The model under review builds one solid part; all positions refer to its coordinate system, in mm. Face numbers are marked on the shaded views. Give positions to 0.01 mm unless a question says otherwise; leave off trailing zeros. Loops run counter-clockwise (first coordinate to the right, second up) from the corner with the lowest first, then second, coordinate; pieces in that order, holes last. Notation, with made-up numbers: M 23,85.5 L 44,85.5 A38 cw 44,123.5 Z; hole C -20,71.5 d10. An arc over 180 degrees is marked long. Write item = value, one per line. Start each with the question number.
1. We need section B-B on y = 0. Give the boundary of the cut face in (x, z).
2. We need section D-D on x = 2.25. Give the boundary of the cut face in (y, z).
3. Draft analysis for pull direction Y (two halves, no side actions). For the marked faces 1, 2, 3 and 4, state which applies: pulls with the +Y half, pulls with the -Y half, needs draft (parallel to the pull), parting line crosses it, or undercut.
4. Wall thickness on line 1 along Y through (x, z) = (-0.5, 0.35); line 2 along Y through (x, z) = (-1.5, 0.7); line 3 along X through (y, z) = (-0.75, 1.3): over which ranges is each line inside the solid? List them lowest first. Write a range as from..to.
5. We need section C-C on x = -1. Give the boundary of the cut face in (y, z), then the cut area to 3 significant figures.
6. We need section A-A on z = 0.15. Give the boundary of the cut face in (x, y) (3 decimals), then the cut area to 3 significant figures.
from build123d import *

# Parameters (mm, degrees)
SKETCH_1_R          = 2
EXTRUDE_542_DEPTH   = 1.7
SKETCH_2_OUTSIDE_W  = 58.042
SKETCH_2_OUTSIDE_H  = 59.068
SKETCH_2_OUTSIDE_R  = 3.5
CUT_EXTRUDE_1_DEPTH = 6.344209483
CUT_EXTRUDE_1_DRAFT = -75


with BuildPart() as part:
    # 草图1 → Extrude 542 (new body)
    with BuildSketch(Plane.XY):
        Polygon((0, 3.83), (-3.316877296, 1.915), (-3.316877296, -1.915), (0, -3.83), (3.316877296, -1.915), (3.316877296, 1.915), align=None)
        Circle(SKETCH_1_R, mode=Mode.SUBTRACT)
    extrude(amount=EXTRUDE_542_DEPTH)


with BuildPart() as cut_extrude_1_tool:
    # 草图2 outside → 切除-拉伸1 (with draft: the straight prism first)
    with BuildSketch(Plane.XY.offset(1.7)):
        Rectangle(SKETCH_2_OUTSIDE_W, SKETCH_2_OUTSIDE_H)
        Circle(SKETCH_2_OUTSIDE_R, mode=Mode.SUBTRACT)
    extrude(amount=-CUT_EXTRUDE_1_DEPTH)
    # 切除-拉伸1: the draft: its side faces are tilted about the plane it starts from
    cut_extrude_1_sides = [cut_extrude_1_tool.faces().sort_by_distance(p)[0] for p in [
        (0, -29.534, -1.472104742),
        (29.021, 0, -1.472104742),
        (0, 29.534, -1.472104742),
        (-29.021, 0, -1.472104742),
        (-3.5, 0, -1.472104742),
    ]]
    draft(cut_extrude_1_sides, Plane.XY.offset(1.7), CUT_EXTRUDE_1_DRAFT)


with BuildPart() as part_1:
    add(part.part)

    # 切除-拉伸1: cut by cut_extrude_1_tool
    add(cut_extrude_1_tool.part, mode=Mode.SUBTRACT)


solid = part_1.part
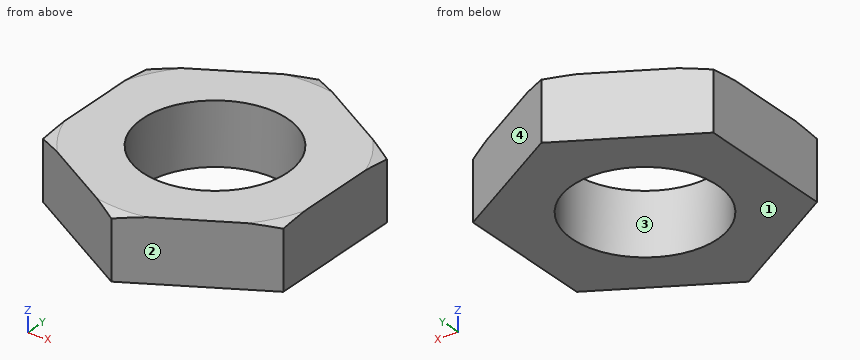
Final values:
q1.outline = M -3.32,0 L -2,0 L -2,1.7 L -3.32,1.7 Z; M 2,0 L 3.32,0 L 3.32,1.7 L 2,1.7 Z
q2.outline = M -2.53,0 L 2.53,0 L 2.53,1.7 L -2.53,1.7 Z
q3.face_1 = needs draft
q3.face_2 = pulls with the -Y half
q3.face_3 = undercut
q3.face_4 = pulls with the +Y half
q4.line_1 = -3.54..-1.94, 1.94..3.54
q4.line_2 = -2.96..-1.32, 1.32..2.96
q4.line_3 = -3.32..-1.85, 1.85..3.32
q5.outline = M -3.25,0 L -1.73,0 L -1.73,1.7 L -3.25,1.7 Z; M 1.73,0 L 3.25,0 L 3.25,1.7 L 1.73,1.7 Z
q5.area = 5.17 mm²
q6.outline = M -3.317,-1.915 L 0,-3.83 L 3.317,-1.915 L 3.317,1.915 L 0,3.83 L -3.317,1.915 Z; hole C 0,0 d4
q6.area = 25.5 mm²
